Autodesk Inventor part; units mm, degrees
ref_plane "YZ Plane" through (0, 0, 0) normal (1, 0, 0) x (0, 1, 0)
ref_plane "XZ Plane" through (0, 0, 0) normal (0, 1, 0) x (-1, 0, 0)
sketch "草图1" plane through (0, 0, 0) normal (0, 1, 0) x (-1, 0, 0)
  circle A0 centre (0, 0) radius 27
  circle A1 centre (0, 0) radius 22.5 construction
  circle A2 centre (22.5, 0) radius 2.5
  circle A3 centre (0, -22.5) radius 2.5
  circle A4 centre (-22.5, 0) radius 2.5
  circle A5 centre (0, 22.5) radius 2.5
  dimension "d0" = 54
  dimension "d1" = 45
  dimension "d2" = 5
  dimension "d3" = 5
  dimension "d4" = 5
  dimension "d5" = 5
extrude "拉伸1" add sketch "草图1" along normal blind 7
sketch "草图2" plane through (0, 7, 0) normal (0, 1, 0) x (1, 0, 0)
  circle A0 centre (0, 0) radius 27
  circle A1 centre (0, 0) radius 10
  dimension "d8" = 20
extrude "拉伸2" add sketch "草图2" along normal blind 12 contours A1
sketch "草图3" plane through (0, 19, 0) normal (0, 1, 0) x (1, 0, 0)
  circle A0 centre (0, 0) radius 10
  circle A1 centre (0, 0) radius 6
  dimension "d11" = 12
extrude "拉伸3" cut sketch "草图3" against normal blind 19 contours A1
sketch "草图4" plane through (0, 0, 0) normal (0, 0, 1) x (1, 0, 0)
  line L0 (10, 19) -> (-10, 19)
  line L1 (-10, 7) -> (10, 7)
  line L2 (27, 7) -> (-27, 7)
  line L3 (-27, 0) -> (27, 0)
  line L4 (8.6752, 19) -> (8.6752, 7)
  line L5 (8.6752, 19) -> (18.2273, 7)
  line L6 (8.6752, 7) -> (18.2273, 7)
  point P0 (0, 0)
extrude "拉伸4" add sketch "草图4" along normal mid plane 6
ref_plane "工作平面1" through (0, 19, 0) normal (-0.866, 0, -0.5) x (0, -1, 0)
sketch "草图5" plane through (0, 19, 0) normal (-0.866, 0, -0.5) x (0, -1, 0)
  point P0 (19, 0)
sketch "草图6" plane through (0, 19, 0) normal (-0.866, 0, -0.5) x (0, -1, 0)
  point P0 (19, 0)
sketch "草图7" plane through (0, 19, 0) normal (-0.866, 0, -0.5) x (0, -1, 0)
  line L0 (12, -2.1716) -> (1.0857, -2.1716)
  ellipse E0 centre (-10.8983, 0) end of major axis (-22.7486, 7.5911) minor radius 7.7307 (1.0857, -7.3678) -> (1.0857, -2.1716) ccw
  line L1 (1.0857, -7.3678) -> (12, -7.3678)
  line L2 (12, -2.1716) -> (12, -7.3678)
  line L3 (0, 10) -> (0, -10)
  line L4 (12, 27) -> (12, -27)
  line L5 (19, -27) -> (19, 27)
  line L6 (0, 8.0111) -> (12, 8.0111)
  line L7 (12, 18.564) -> (0, 8.0111)
  line L8 (12, 18.564) -> (12, 8.0111)
  point P0 (19, 0)
extrude "拉伸5" add sketch "草图7" along normal mid plane 6 contours L6 L7 L4
ref_plane "工作平面2" through (0, 19, 0) normal (0.866, 0, -0.5) x (0, -1, 0)
sketch "草图8" plane through (0, 19, 0) normal (0.866, 0, -0.5) x (0, -1, 0)
  line L0 (0, 10) -> (0, -10)
  line L1 (12, -2.1716) -> (1.7379, -2.1716)
  ellipse E0 centre (-9.1096, 0) end of major axis (1.2979, -8.0654) minor radius 7.4792 (1.7379, -7.3678) -> (1.7379, -2.1716) ccw
  line L2 (1.7379, -7.3678) -> (12, -7.3678)
  line L3 (12, -7.3678) -> (12, -7.3678)
  line L4 (12, -7.3678) -> (1.0857, -7.3678)
  ellipse E1 centre (-10.8983, 0) end of major axis (-22.7486, 7.5911) minor radius 7.7307 (1.0857, -7.3678) -> (1.0857, -2.1716) ccw
  line L5 (1.0857, -2.1716) -> (12, -2.1716)
  line L6 (12, -2.1716) -> (12, -2.1716)
  line L7 (12, 27) -> (12, -27)
  line L8 (19, -27) -> (19, 27)
  line L9 (0, 6.3008) -> (12, 6.3008)
  line L10 (0, 6.3008) -> (12, 15.6151)
  line L11 (12, 15.6151) -> (12, 6.3008)
  point P0 (19, 0)
extrude "拉伸6" add sketch "草图8" along normal mid plane 6 contours L9 L10 L7
Source: CAD feature listing. Evaluate the final solid. Frame: model axes, mm. A direction names the side the tool comes from. Coordinates: 2 decimals unless noted, no trailing zeros. Write each loop counter-clockwise with the first axis right and the second up, starting at its lowest first coordinate (ties: lowest second). Pieces come first, ordered by that corner, then holes. Notation, with made-up numbers: (65.5, -14) -> (72.5, -14) arc R20 cw to (72.5, -4) -> close; hole circle Ø6 at (19, 40). An arc over 180 degrees is marked (long way). Return JSON: item names as keys, results as strings. Group by question number.
1) Ray query, line 1 along Z through (x, y) = (0, 2); line 2 along X through (y, z) = (7.25, 2); line 3 along Y through (x, z) = (3, -14). Return the intervals inside material, ascending.
2) Section query B-B, the plane z = 22.5. Return loops of the section in (x, y), plus the area to 3 significant figures.
3) Section query D-D, the plane x = 22.5. Return loops of the section in (y, z), plus the area to 3 significant figures.
4) Mould query, pull axis Z, two halves, no side actions, for faces 1 (the face through (-8.653, 9.922, 8.987)), 2 (the face through (4.614, 12.916, -8.872)), 3 (the face through (5.85, 3.45, 26.36)), 4 (the face through (0.4, 0, 6.4)). Classes: +Z half, -Z half, draft (parallel to the pull), parting line (faces both ways), or undercut.
5) Contact query for flat-ended pins moving along their axis: P1, Ø8, axis at y = 2, z = -18, coming from the -X side; P2, Ø11, axis at x = 0, z = 0, coming from the -Y side; P3, Ø7, axis at x = 14.5, y = 11.5, coming from the -Z side; P4, Ø7, axis at x = 15, y = 14, coming from the +Z side. Output: stop coordinate, or through.
6) Section query C-C, the plane y = 11.25. Return loops of the section in (x, z).
7) Set-up query: faces 5 (the face through (-6.304, 10.969, -10.834)), 6 (the face through (12, 10, 3)), 7 (the face through (-12, 7, 0)), 8 (the face through (-8.233, 9.229, -8.26)). Return all of +Z, -Z, +X, -X, +Y, -Y with unobstructed straight access to the full face (end or side cutting, diameter ignored); none if empty.
8) Section query A-A, the plane x = 0. Return loops of the section in (y, z).
From the geometry:
{
 "1": {"line 1": "-27 to -25, -20 to -6, 6 to 20, 25 to 27", "line 2": "-9.8 to -5.66, 5.66 to 18.03", "line 3": "0 to 7"},
 "2": {"outline": "(-14.92, 0) -> (-2.5, 0) -> (-2.5, 7) -> (-14.92, 7) -> close; (2.5, 0) -> (14.92, 0) -> (14.92, 7) -> (2.5, 7) -> close", "area": "174 mm²"},
 "3": {"outline": "(0, -14.92) -> (7, -14.92) -> (7, -2.5) -> (0, -2.5) -> close; (0, 2.5) -> (7, 2.5) -> (7, 14.92) -> (0, 14.92) -> close", "area": "174 mm²"},
 "4": {"face 1": "undercut", "face 2": "undercut", "face 3": "parting line", "face 4": "draft"},
 "5": {"P1": "x = -23.09", "P2": "through", "P3": "z = -3", "P4": "z = 3"},
 "6": {"outline": "(-10.01, 11.34) -> (-7.37, 6.76) arc R10 ccw to (-7.37, -6.76) -> (-8.76, -9.17) -> (-3.56, -12.17) -> (-2.17, -9.76) arc R10 ccw to (9.54, -3) -> (14.84, -3) -> (14.84, 3) -> (9.54, 3) arc R10 ccw to (-2.17, 9.76) -> (-4.82, 14.34) -> close; hole circle Ø12 at (0, 0)"},
 "7": {"face 5": "-Z, -X, +Y", "face 6": "+Z, +X, +Y", "face 7": "+Y", "face 8": "-X, +Y"},
 "8": {"outline": "(0, -27) -> (7, -27) -> (7, -25) -> (0, -25) -> close; (0, -20) -> (7, -20) -> (7, -10) -> (19, -10) -> (19, -6) -> (0, -6) -> close; (0, 6) -> (19, 6) -> (19, 10) -> (7, 10) -> (7, 20) -> (0, 20) -> close; (0, 25) -> (7, 25) -> (7, 27) -> (0, 27) -> close"}
}
